Could you check a few things on this drawing? It's one solid part, dimensions in mm from its lowest x, y, z. Coordinates: 2 decimals unless noted, no trailing zeros. Order: outer loops, then holes, each group sorted by start corner. A loop starts at its lowest first (then second) coordinate and runs counter-clockwise, first axis right, second up. Notation, with made-up numbers: (-8, 39.25) -> (28, 39.25) arc R21 cw to (28, 73.25) -> close; hole circle Ø6 at (35, 72.5). An arc over 180 degrees is marked (long way). Answer as CSV lines item,"result".
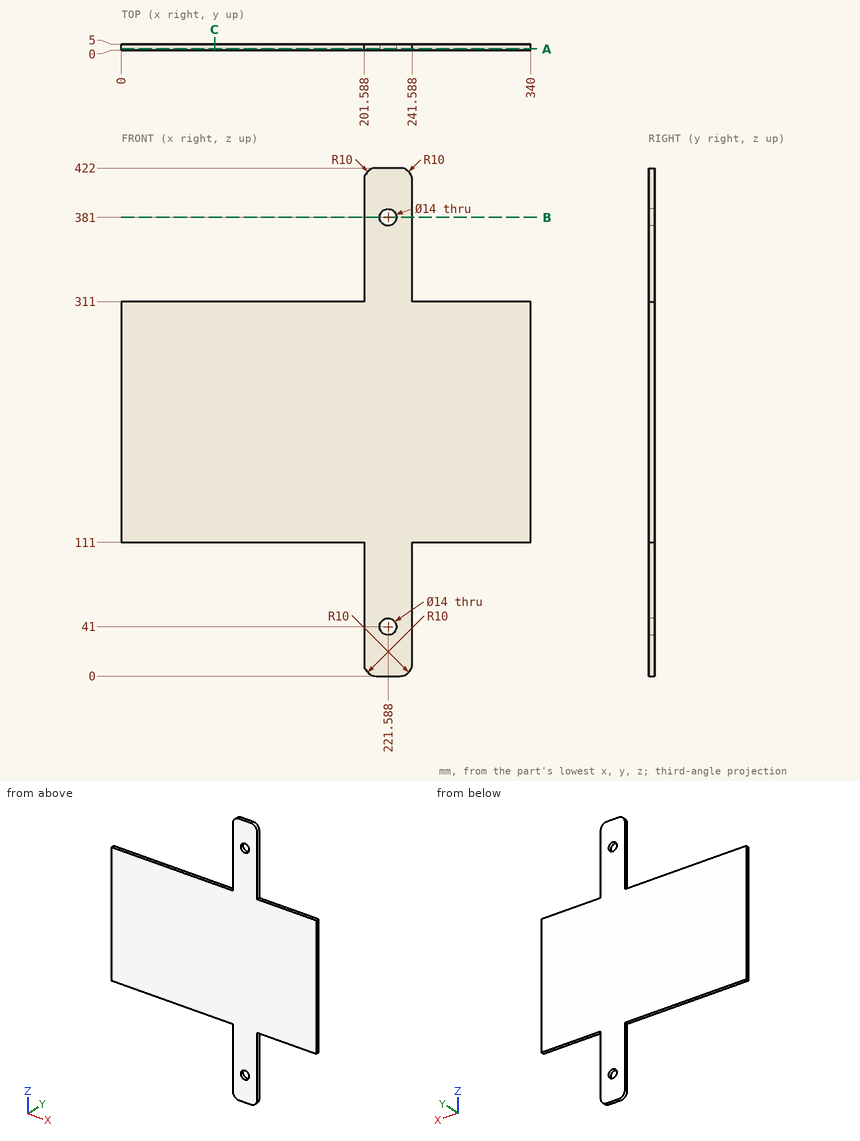
Q1. Imagine slicing it at A-A (y = 0.85). List the corners of the cut face in (x, z) for me, and give its area (3 significant figures).
Solution:
outline,"(0, 111) -> (201.59, 111) -> (201.59, 10) arc R10 ccw to (211.59, 0) -> (231.59, 0) arc R10 ccw to (241.59, 10) -> (241.59, 111) -> (340, 111) -> (340, 311) -> (241.59, 311) -> (241.59, 412) arc R10 ccw to (231.59, 422) -> (211.59, 422) arc R10 ccw to (201.59, 412) -> (201.59, 311) -> (0, 311) -> close; hole circle Ø14 at (221.59, 41); hole circle Ø14 at (221.59, 381)"
area,"76,500 mm2"
Q2. For P1, Ø8, axis at x = 279, z = 208, coming from the -Y side; P2, Ø1, axis at x = 268.5, y = 3.5, coming from the +Z side; P3, Ø2.5, axis at y = 2, z = 382.5, coming from the -X side; P4, Ø1.5, axis at x = 56, y = 3.5, coming from the -Z side, each with a flat end and sliding along its axis, tell me the tip position at first contact or that it passes through.
Solution:
P1,"y = 0"
P2,"z = 311"
P3,"x = 201.59"
P4,"z = 111"
Q3. If I drill on line 1 (Z direction, x = 222, y = 0.5); line 2 (X direction, y = 1.6, z = 381); line 3 (Z direction, x = 200, y = 1.75), over which ranges is the centre line in solid material (lowest first)?
Solution:
line 1,"0 to 34.01, 47.99 to 374.01, 387.99 to 422"
line 2,"201.59 to 214.59, 228.59 to 241.59"
line 3,"111 to 311"
Q4. Imagine slicing it at B-B (z = 381). List the corners of the cut face in (x, y) for me, and give its area (3 significant figures).
Solution:
outline,"(201.59, 0) -> (214.59, 0) -> (214.59, 5) -> (201.59, 5) -> close; (228.59, 0) -> (241.59, 0) -> (241.59, 5) -> (228.59, 5) -> close"
area,"130 mm2"
Q5. Imagine slicing it at C-C (x = 77.5). List the corners of the cut face in (y, z) for me.
Solution:
outline,"(0, 111) -> (5, 111) -> (5, 311) -> (0, 311) -> close"
